from build123d import *

# Parameters (mm, degrees)
SKETCH1_W           = 114.3
SKETCH1_H           = 114.3
SKETCH1_W_2         = 101.6
SKETCH1_H_2         = 101.6
EXTRUDE_THIN1_DEPTH = 50.8
SKETCH3_W           = 114.3
SKETCH3_H           = 114.3
SKETCH3_W_2         = 101.6
SKETCH3_H_2         = 101.6
EXTRUDE_THIN2_DEPTH = 50.8
BOSS_EXTRUDE1_DEPTH = 114.3
BOSS_EXTRUDE2_REACH = 165.011
SKETCH5_W           = 6.35
SKETCH5_H           = 101.6
SKETCH6_R           = 6.35
CUT_EXTRUDE1_DEPTH  = 224.426173489


with BuildPart() as part:
    # Sketch1 → Extrude-Thin1 (new body)
    with BuildSketch(Plane.XY):
        Rectangle(SKETCH1_W, SKETCH1_H)
        Rectangle(SKETCH1_W_2, SKETCH1_H_2, mode=Mode.SUBTRACT)
    extrude(amount=EXTRUDE_THIN1_DEPTH)

    # Sketch3 → Extrude-Thin2 (add)
    with BuildSketch(Plane(origin=(57.15, 0, 0), x_dir=(0, 0, -1), z_dir=(1, 0, 0))):
        with Locations((-101.6, 0)):
            Rectangle(SKETCH3_W, SKETCH3_H)
        with Locations((-101.6, 0)):
            Rectangle(SKETCH3_W_2, SKETCH3_H_2, mode=Mode.SUBTRACT)
    extrude(amount=EXTRUDE_THIN2_DEPTH)

    # Sketch4 → Boss-Extrude1 (add)
    with BuildSketch(Plane.ZY.offset(-57.15)):
        Polygon((50.8, -50.8), (50.8, -57.15), (158.75, -57.15), (158.75, 57.15), (50.8, 57.15), (50.8, 50.8), (152.4, 50.8), (152.4, -50.8), align=None)
    extrude(amount=BOSS_EXTRUDE1_DEPTH)

    # Sketch5 → Boss-Extrude2 (add, up to next)
    with BuildSketch(Plane.XY.offset(50.8), mode=Mode.PRIVATE) as boss_extrude2_sk1:
        with Locations((-53.975, 0)):
            Rectangle(SKETCH5_W, SKETCH5_H)
    boss_extrude2_tool1 = extrude(boss_extrude2_sk1.sketch, amount=BOSS_EXTRUDE2_REACH, mode=Mode.PRIVATE) - part.part
    add(boss_extrude2_tool1.solids().sort_by_distance((-53.975, 0, 50.8))[0])

    # Sketch6 → Cut-Extrude1 (cut, through all)
    with BuildSketch(Plane(origin=(0, 57.15, 0), x_dir=(1, 0, 0), z_dir=(0, 1, 0))):
        with Locations(Location((0, -50.8, 0), (0, 0, 270))):
            Circle(SKETCH6_R)
    cut_extrude1 = extrude(amount=-CUT_EXTRUDE1_DEPTH, mode=Mode.SUBTRACT)

    # Mirror1: Cut-Extrude1 across plane
    add(cut_extrude1.mirror(Plane(origin=(50.8, 0, 50.8), x_dir=(-0.7071067811865477, 0, 0.7071067811865474), z_dir=(0.7071067811865476, 0, 0.7071067811865476))), mode=Mode.SUBTRACT)


solid = part.part
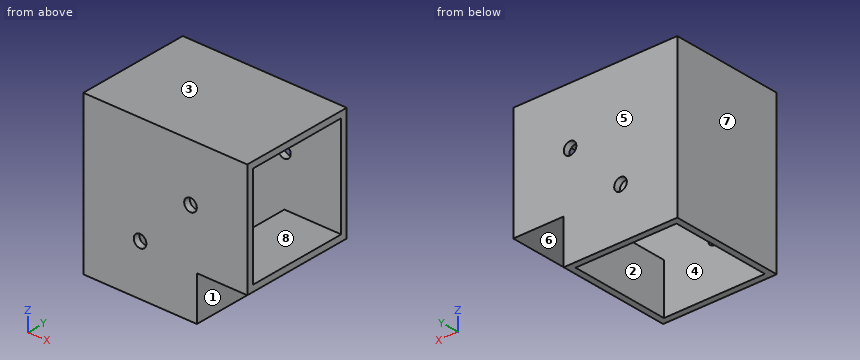
The model under review builds one solid part; all positions refer to its coordinate system, in mm. Face numbers are marked on the shaded views. A direction names the side the tool comes from. Coordinates: 2 decimals unless noted, no trailing zeros. Write each loop counter-clockwise with the first axis right and the second up, starting at its lowest first coordinate (ties: lowest second). Pieces come first, ordered by that corner, then holes. Notation, with made-up numbers: (-14.5, 53) -> (16.5, 53) arc R25 ccw to (16.5, 79) -> close; hole circle Ø7 at (-9.75, -10.75). An arc over 180 degrees is marked (long way). Answer in a Markdown table with one row per item.
1. We need section D-D, the plane x = 0. State the section outline as (y, z) points.
Answers below:
| item | result |
|---|---|
| outline | (-57.15, 0) -> (-50.8, 0) -> (-50.8, 44.45) -> (-57.15, 44.45) -> close; (-57.15, 57.15) -> (-50.8, 57.15) -> (-50.8, 152.4) -> (50.8, 152.4) -> (50.8, 57.15) -> (57.15, 57.15) -> (57.15, 158.75) -> (-57.15, 158.75) -> close; (50.8, 0) -> (57.15, 0) -> (57.15, 44.45) -> (50.8, 44.45) -> close |
2. For the marked faces 4, 5, 6, 7 and 8, list the 3-axis set-ups (+Z, -Z, +X, -X, +Y, -Y) from which the entire face can be reached by the end or side of a thin tool; tool diameter is ignored.
Answers below:
| item | result |
|---|---|
| face 4 | none |
| face 5 | +Z, -Z, +X, -X, +Y |
| face 6 | -Z, +X, +Y, -Y |
| face 7 | +Z, -Z, -X, +Y, -Y |
| face 8 | +X |
3. Draft analysis for pull direction X (two halves, no side actions). For the marked faces 1, 2 and 3, state which applies: +X half, -X half, draft (parallel to the pull), parting line (faces both ways), or undercut.
Answers below:
| item | result |
|---|---|
| face 1 | +X half |
| face 2 | undercut |
| face 3 | draft |
4. We need section B-B, the plane z = 101.6. State the section outline as (x, y) points.
Answers below:
| item | result |
|---|---|
| outline | (-57.15, -57.15) -> (44.45, -57.15) -> (44.45, -50.8) -> (-50.8, -50.8) -> (-50.8, 50.8) -> (44.45, 50.8) -> (44.45, 57.15) -> (-57.15, 57.15) -> close; (57.15, -57.15) -> (107.95, -57.15) -> (107.95, -50.8) -> (57.15, -50.8) -> close; (57.15, 50.8) -> (107.95, 50.8) -> (107.95, 57.15) -> (57.15, 57.15) -> close |
5. Clearance check with flat-ended pins moving along their axes: pin 1 Ø12 at (y, z) = (-38.5, 19.5) entering from +X; pin 2 Ø10 at (y, z) = (5.5, 73.5) entering from +X; pin 3 Ø8 at (x, y) = (88.5, 7) entering from -Z. State where each tip first meets the part, or that it passes through.
Answers below:
| item | result |
|---|---|
| pin 1 | stops at x = 57.15 |
| pin 2 | stops at x = -50.8 |
| pin 3 | stops at z = 44.45 |
6. Wall thickness on probe 1 along Y at (x, z) = (-8.5, 73.5); probe 2 along Z at (x, y) = (50.8, -54); probe 3 along X at (y, z) = (55.25, 50.8): over which ranges is each line inside the solid? List them lowest first. Write a range as [from, to].
Answers below:
| item | result |
|---|---|
| probe 1 | y = [-57.15, -50.8], [50.8, 57.15] |
| probe 2 | z = [0, 95.25], [107.95, 158.75] |
| probe 3 | x = [-57.15, -6.35], [6.35, 107.95] |
7. We need section A-A, the plane x = 82. State the section outline as (y, z) points, and give its area (3 significant figures).
Answers below:
| item | result |
|---|---|
| outline | (-57.15, 44.45) -> (57.15, 44.45) -> (57.15, 158.75) -> (-57.15, 158.75) -> close; hole (-50.8, 50.8) -> (50.8, 50.8) -> (50.8, 152.4) -> (-50.8, 152.4) -> close |
| area | 2,740 mm^2 |
8. We need section C-C, the plane y = 23. State the section outline as (x, z) points.
Answers below:
| item | result |
|---|---|
| outline | (-57.15, 0) -> (-50.8, 0) -> (-50.8, 152.4) -> (107.95, 152.4) -> (107.95, 158.75) -> (-57.15, 158.75) -> close; (50.8, 0) -> (57.15, 0) -> (57.15, 44.45) -> (107.95, 44.45) -> (107.95, 50.8) -> (50.8, 50.8) -> close |
